For this review, take the finished solid that the model builds, in its own axes (mm). Coordinates: 2 decimals unless noted, no trailing zeros. Order: outer loops, then holes, each group sorted by start corner. A loop starts at its lowest first (then second) coordinate and runs counter-clockwise, first axis right, second up.
from build123d import *


with BuildPart() as f3:
    # F0 (on Top) → F3 section 0
    with BuildSketch(Plane.XY, mode=Mode.PRIVATE) as f3_s0:
        Polygon((137.427947, 6.804655), (115.613766, 74.606977), (62.82097, 122.418421), (-6.804655, 137.427947), (-74.606977, 115.613766), (-122.418421, 62.82097), (-137.427947, -6.804655), (-115.613766, -74.606977), (-62.82097, -122.418421), (6.804655, -137.427947), (74.606977, -115.613766), (122.418421, -62.82097), align=None)
    loft([Vertex(10.073566, 40.029168, 152.4), f3_s0.sketch])


solid = f3.part
1. Clearance check with flat-ended pins moving along their axes: pin 1 Ø1 at (x, z) = (-32.5, 20.5) entering from +Y; pin 2 Ø10 at (y, z) = (7, 58) entering from -X; pin 3 Ø6 at (y, z) = (-32, 55.5) entering from -X. State where each tip first meets the part, or that it passes through.
Answer below:
pin 1: stops at y = 115.7
pin 2: stops at x = -85.57
pin 3: stops at x = -73.46
2. To check wall thickness, follow L1, parallel to Z at x = 93.5, y = 29.5; L2, parallel to Y at x = 30.5, z = 84; L3, parallel to Y at x = 14.5, z = 31.5. State the ranges of each line that lie inside material, in increasing order.
Answer below:
L1: z = 0 to 47.84
L2: y = -32.57 to 77.71
L3: y = -98.49 to 113.46
3. Take a section at A-A, the plane z = 119. Give the boundary of the cut face in (x, y), plus the area to 3 significant figures.
Answer below:
outline: (-22.25, 29.77) - (-17.47, 14.91) - (-5.9, 4.43) - (9.36, 1.14) - (24.22, 5.92) - (34.7, 17.49) - (37.98, 32.75) - (33.2, 47.61) - (21.63, 58.09) - (6.37, 61.38) - (-8.49, 56.59) - (-18.96, 45.02) - close
area: 2,730 mm2
4. Take a section at D-D, the plane z = 65. Give the boundary of the cut face in (x, y).
Answer below:
outline: (-74.52, 13.17) - (-62.01, -25.71) - (-31.73, -53.13) - (8.2, -61.74) - (47.08, -49.23) - (74.5, -18.95) - (83.11, 20.98) - (70.6, 59.86) - (40.32, 87.28) - (0.39, 95.89) - (-38.49, 83.38) - (-65.91, 53.1) - close
5. Take a section at C-C, the plane y = -47. Give the boundary of the cut face in (x, z), plus the area to 3 significant figures.
Answer below:
outline: (-124.5, 0) - (125.83, 0) - (105.14, 23.44) - (46.16, 67.18) - (8.47, 77.66) - (-28.98, 70.75) - (-85.35, 36.7) - close
area: 12,200 mm2
6. The part is to be moulded in two halves that separate along X. For faces 1 (the face through (2, 2, 0)), 2 (the face through (78.627, -49.736, 41.267)), 3 (the face through (-77.27, 28.83, 58.2)), say which applies: +X half, -X half, draft (parallel to the pull), parting line (faces both ways), or undercut.
Answer below:
face 1: draft
face 2: +X half
face 3: -X half
7. Take a section at B-B, the plane x = 31. Give the boundary of the cut face in (y, z), plus the area to 3 significant figures.
Answer below:
outline: (-129.64, 0) - (129.28, 0) - (72.72, 91.94) - (46.89, 122.18) - (34.57, 127.36) - (20.87, 124.01) - (-10.44, 102.98) - close
area: 18,300 mm2
